Can you work these out from the model? Positions are in its coordinate system, mm. A direction names the side the tool comes from. Round coordinates to 2 decimals unless told otherwise and drop trailing zeros. Write each loop counter-clockwise with the first axis right and the second up, starting at its lowest first coordinate (ties: lowest second). Pieces come first, ordered by that corner, then holes. Notation, with made-up numbers: (66.25, -33.5) -> (75.25, -33.5) arc R7 cw to (75.25, -21.5) -> close; hole circle Ø4 at (-0.5, -8.5). An arc over 180 degrees is marked (long way). Use CSV: the item, a comma, the result in double quotes.
```python
from build123d import *

# Parameters (mm, degrees)
F0_R     = 31.75
F1_DEPTH = 6.35
F2_W     = 6.35
F2_H     = 25.399766
F3_DEPTH = 44.45


with BuildPart() as f1:
    # F0 (on Right) → F1 (new body)
    with BuildSketch(Plane.YZ):
        with BuildLine():
            ThreePointArc((37.479318, 6.849139), (33.890578, 17.408007), (27.398215, 26.475419))
            ThreePointArc((27.398215, 26.475419), (-37.580446, 6.270574), (17.318016, -33.936652))
            ThreePointArc((17.318016, -33.936652), (24.856502, -28.874977), (30.983175, -22.173246))
            ThreePointArc((30.983175, -22.173246), (36.27719, -11.64369), (38.1, 0))
            ThreePointArc((38.1, 0), (37.944512, 3.438602), (37.479318, 6.849139))
        make_face()
        Circle(F0_R, mode=Mode.SUBTRACT)
        with BuildLine():
            ThreePointArc((38.083032, 6.349766), (37.691291, 6.490788), (37.479318, 6.849139))
            ThreePointArc((37.479318, 6.849139), (37.944512, 3.438602), (38.1, 0))
            ThreePointArc((38.1, 0), (36.27719, -11.64369), (30.983175, -22.173246))
            ThreePointArc((30.983175, -22.173246), (34.214004, -19.86517), (38.1, -19.05))
            Line((38.1, -19.05), (44.45, -19.05))
            Line((44.45, -19.05), (44.45, 6.349766))
            Line((44.45, 6.349766), (38.083032, 6.349766))
        make_face()
    extrude(amount=F1_DEPTH)

    # F2 (on face) → F3 (join)
    with BuildSketch(Plane.YZ.offset(6.35)):
        with Locations((41.275, -6.350117)):
            Rectangle(F2_W, F2_H)
    extrude(amount=F3_DEPTH)

    # F4: F1 across face


with BuildPart() as f1_1:
    add(f1.part)
    add(f1.part.mirror(Plane(origin=(50.8, 41.275, -6.350117), x_dir=(0, 1, 0), z_dir=(1, 0, 0))))


solid = f1_1.part
```
Q1. Suppose I cut it at B-B (z = 0). Write out the boundary of the cut face in (x, y).
Resolved:
outline,"(0, -38.1) -> (6.35, -38.1) -> (6.35, -31.75) -> (0, -31.75) -> close; (0, 31.75) -> (6.35, 31.75) -> (6.35, 38.1) -> (95.25, 38.1) -> (95.25, 31.75) -> (101.6, 31.75) -> (101.6, 44.45) -> (0, 44.45) -> close; (95.25, -38.1) -> (101.6, -38.1) -> (101.6, -31.75) -> (95.25, -31.75) -> close"
Q2. Please list where these lines run through material, in increasing order: probe 1 along Z at (x, y) = (98.5, 0); probe 2 along X at (y, z) = (-31, -9); probe 3 along Y at (x, z) = (56.5, -8).
Resolved:
probe 1,"z = -38.1 to -31.75, 31.75 to 38.1"
probe 2,"x = 0 to 6.35, 95.25 to 101.6"
probe 3,"y = 38.1 to 44.45"
Q3. Suppose I cut it at C-C (z = 23). Write out the boundary of the cut face in (x, y).
Resolved:
outline,"(0, -30.37) -> (6.35, -30.37) -> (6.35, -21.89) -> (0, -21.89) -> close; (0, 21.89) -> (6.35, 21.89) -> (6.35, 30.37) -> (0, 30.37) -> close; (95.25, -30.37) -> (101.6, -30.37) -> (101.6, -21.89) -> (95.25, -21.89) -> close; (95.25, 21.89) -> (101.6, 21.89) -> (101.6, 30.37) -> (95.25, 30.37) -> close"
Q4. If we mould it in two halves opening along X, with no side actions, what happens to faces 1 (the face through (0, 27, -17)), 2 (the face through (51, 38.1, -7)), 3 (the face through (52, 44.45, -7))? For each: released by +X, released by -X, zero draft, split by the parting line, or undercut.
Resolved:
face 1,"released by -X"
face 2,"undercut"
face 3,"zero draft"
Q5. Will these pins go through, and if not, where does the flat tip stop? P1, Ø1.5, axis at x = 24, z = -6.5, coming from the -Y side; P2, Ø7, axis at x = 41, y = 39.5, coming from the +Z side; P3, Ø5, axis at x = 40.5, y = 42, coming from the -Z side.
Resolved:
P1,"stops at y = 38.1"
P2,"stops at z = 6.35"
P3,"stops at z = -19.05"
Q6. On a 3-axis mill with a long thin cutter (end or side, diameter ignored), from which of +Z, -Z, +X, -X, +Y, -Y can I reach the whole of each face in a straight line? I mean faces 4 (the face through (98.47, 34.16, -19.89)), 5 (the face through (6.35, 22.4, 22.8)). Say none if no direction works.
Resolved:
face 4,"-Z, +X, -X, +Y"
face 5,"+Z, -Z, -Y"
Q7. Suppose I cut it at A-A (y = 0). Write out the boundary of the cut face in (x, z), and give its area (3 significant figures).
Resolved:
outline,"(0, -38.1) -> (6.35, -38.1) -> (6.35, -31.75) -> (0, -31.75) -> close; (0, 31.75) -> (6.35, 31.75) -> (6.35, 38.1) -> (0, 38.1) -> close; (95.25, -38.1) -> (101.6, -38.1) -> (101.6, -31.75) -> (95.25, -31.75) -> close; (95.25, 31.75) -> (101.6, 31.75) -> (101.6, 38.1) -> (95.25, 38.1) -> close"
area,"161 mm^2"
Q8. Suppose I cut it at D-D (y = 34.5). Write out the boundary of the cut face in (x, z), and give its area (3 significant figures).
Resolved:
outline,"(0, -19.75) -> (6.35, -19.75) -> (6.35, 16.17) -> (0, 16.17) -> close; (95.25, -19.75) -> (101.6, -19.75) -> (101.6, 16.17) -> (95.25, 16.17) -> close"
area,"456 mm^2"
